Input: part model. Units: mm. Frame: model coordinates. Face numbers are marked on the shaded views. A direction names the side the tool comes from. Coordinates: 2 decimals unless noted, no trailing zeros. Order: outer loops, then holes, each group sorted by start corner. A loop starts at its lowest first (then second) coordinate and runs counter-clockwise, first axis right, second up.
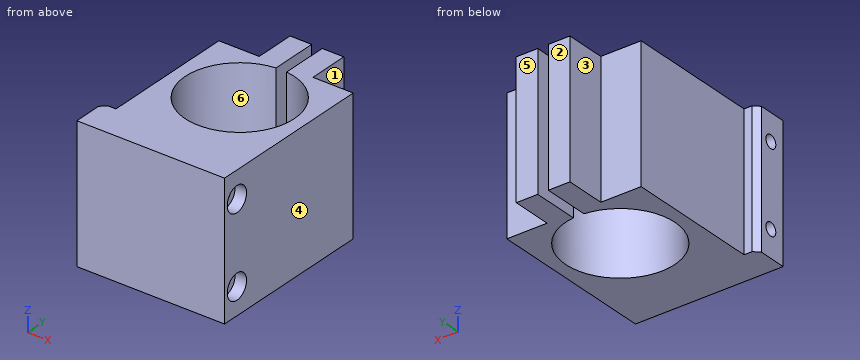
from build123d import *

# Parameters (mm, degrees)
BOSS_EXTRUDE1_DEPTH                            = 25.4
CHAMFER1_SIZE                                  = 1
CBORE_FOR_2_SOCKET_HEAD_CAP_SCREW1_D           = 2.4384
CBORE_FOR_2_SOCKET_HEAD_CAP_SCREW1_CBORE_D     = 4.7625
CBORE_FOR_2_SOCKET_HEAD_CAP_SCREW1_CBORE_DEPTH = 2.1844


with BuildPart() as part:
    # Sketch1 → Boss-Extrude1 (new body)
    with BuildSketch(Plane.XY):
        with BuildLine():
            Line((0.109825555, 12.7), (0.109825555, 6.35))
            Line((0.109825555, 6.35), (28.049825555, 6.35))
            Line((28.049825555, 6.35), (28.049825555, 38.1))
            Line((28.049825555, 38.1), (20.429825555, 38.1))
            Line((20.429825555, 38.1), (20.429825555, 45.72))
            Line((20.429825555, 45.72), (16.349825555, 45.72))
            Line((16.349825555, 45.72), (16.349825555, 36.933800162))
            ThreePointArc((16.349825555, 36.933800162), (15.349825555, 16.3576), (14.349825555, 36.933800162))
            Line((14.349825555, 36.933800162), (14.349825555, 45.72))
            Line((14.349825555, 45.72), (10.269825555, 45.72))
            Line((10.269825555, 45.72), (10.269825555, 38.1))
            Line((10.269825555, 38.1), (2.649825555, 38.1))
            Line((2.649825555, 38.1), (2.649825555, 12.7))
            Line((2.649825555, 12.7), (0.109825555, 12.7))
        make_face()
    extrude(amount=BOSS_EXTRUDE1_DEPTH)

    # Chamfer1
    chamfer1_edges = [part.edges().sort_by_distance(p)[0] for p in [
        (0.109825555, 12.7, 12.7),
    ]]
    chamfer(chamfer1_edges, length=CHAMFER1_SIZE)

    # CBORE for #2 Socket Head Cap Screw1 (through all)
    with Locations(Plane(origin=(28.049825555, 0, 0), x_dir=(0, 0, -1), z_dir=(1, 0, 0))):
        with Locations((-20.32, 9.398), (-5.08, 9.398)):
            CounterBoreHole(CBORE_FOR_2_SOCKET_HEAD_CAP_SCREW1_D / 2, CBORE_FOR_2_SOCKET_HEAD_CAP_SCREW1_CBORE_D / 2, CBORE_FOR_2_SOCKET_HEAD_CAP_SCREW1_CBORE_DEPTH)


solid = part.part
Item 1: Draft query along X for the marked faces 4, 5 and 6. Return one class per face: pulls with the +X half, pulls with the -X half, needs draft (parallel to the pull), parting line crosses it, or undercut.
Response values:
face 4: pulls with the +X half
face 5: needs draft
face 6: undercut
Item 2: Cut plane D-D on z = 13.5. Return loops of the section in (x, y).
Response values:
outline: (0.11, 6.35) - (28.05, 6.35) - (28.05, 38.1) - (20.43, 38.1) - (20.43, 45.72) - (16.35, 45.72) - (16.35, 36.93) arc R10.31 cw (long way) to (14.35, 36.93) - (14.35, 45.72) - (10.27, 45.72) - (10.27, 38.1) - (2.65, 38.1) - (2.65, 12.7) - (1.11, 12.7) - (0.11, 11.7) - close
Item 3: Ray query, probe 1 along Z at (x, y) = (20.75, 10); probe 2 along X at (y, z) = (40.5, 16.75); probe 3 along Y at (x, z) = (27.65, 20.32). Return the intervals inside material, ascending.
Response values:
probe 1: z = 0 to 4.02, 6.14 to 19.26, 21.38 to 25.4
probe 2: x = 10.27 to 14.35, 16.35 to 20.43
probe 3: y = 6.35 to 7.02, 11.78 to 38.1
Item 4: Pin query (flat end, axial travel): pin 1 Ø4.5 at (y, z) = (41.5, 7) entering from +X; pin 2 Ø8.5 at (y, z) = (41, 17) entering from -X; pin 3 Ø4 at (x, z) = (7, 18.5) entering from +Y. Return the tip coordinate at first contact, or that it passes through.
Response values:
pin 1: stops at x = 20.43
pin 2: stops at x = 2.65
pin 3: stops at y = 38.1
Item 5: Cut plane A-A on x = 9.25. Return loops of the section in (y, z).
Response values:
outline: (6.35, 0) - (18.36, 0) - (18.36, 25.4) - (6.35, 25.4) - close; (34.98, 0) - (38.1, 0) - (38.1, 25.4) - (34.98, 25.4) - close; hole circle Ø2.44 at (9.4, 5.08); hole circle Ø2.44 at (9.4, 20.32)
Item 6: Cut plane B-B on z = 20.32. Return loops of the section in (x, y), then the cut area to 3 significant figures.
Response values:
outline: (0.11, 6.35) - (28.05, 6.35) - (28.05, 7.02) - (25.87, 7.02) - (25.87, 8.18) - (0.11, 8.18) - close; (0.11, 10.62) - (25.87, 10.62) - (25.87, 11.78) - (28.05, 11.78) - (28.05, 38.1) - (20.43, 38.1) - (20.43, 45.72) - (16.35, 45.72) - (16.35, 36.93) arc R10.31 cw (long way) to (14.35, 36.93) - (14.35, 45.72) - (10.27, 45.72) - (10.27, 38.1) - (2.65, 38.1) - (2.65, 12.7) - (1.11, 12.7) - (0.11, 11.7) - close
area: 475 mm2
Item 7: Access query for the marked faces 1, 2 and 3. Directions: +Z, -Z, +X, -X, +Y, -Y. A direction counts if a zero-diameter tool reaches every point of the face in a straight line with its end or side. Return the directions, or none.
Response values:
face 1: +Z, -Z, +X, +Y
face 2: +Z, -Z, +X, -X, +Y
face 3: +Z, -Z, -X, +Y
Item 8: Cut plane C-C on y = 26.67. Return loops of the section in (x, z), then the cut area to 3 significant figures.
Response values:
outline: (2.65, 0) - (5.04, 0) - (5.04, 25.4) - (2.65, 25.4) - close; (25.66, 0) - (28.05, 0) - (28.05, 25.4) - (25.66, 25.4) - close
area: 121 mm2
